Study the drawing (mm; zero at the part's minimum x, y, z) and answer. A direction names the side the tool comes from. Round coordinates to 2 decimals unless told otherwise and drop trailing zeros. Loops run counter-clockwise (first coordinate to the right, second up) from the corner with the lowest first, then second, coordinate; pieces in that order, holes last. Notation, with made-up numbers: (17.25, 24.5) -> (75.25, 24.5) arc R12 cw to (75.25, 38.5) -> close; hole circle Ø10 at (6.5, 56.25). An arc over 180 degrees is marked (long way). Use one line per item in the form item = value.
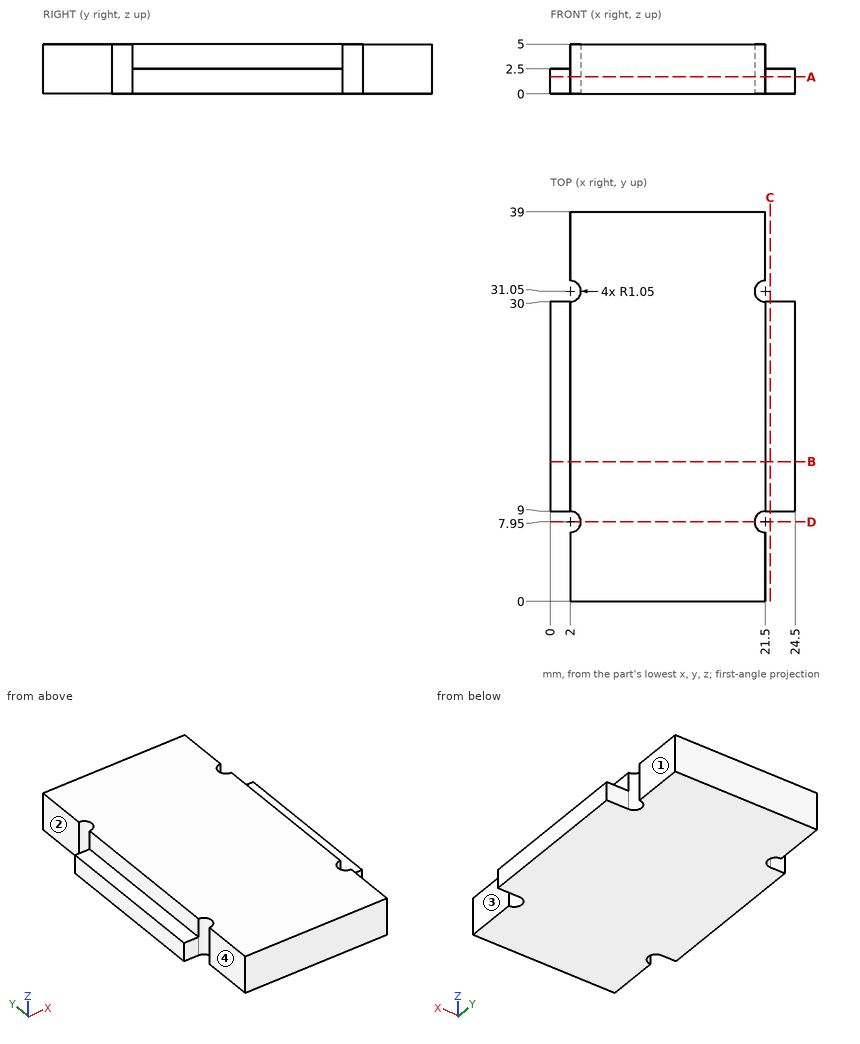
(1) Find section D-D, the plane y = 7.95. Write down the section's boundary in (x, z), then the cut area to 3 significant figures.
Completed:
outline = (3.05, 0) -> (20.45, 0) -> (20.45, 5) -> (3.05, 5) -> close
area = 87.0 mm2
(2) Given P1, Ø12, axis at x = 5.5, y = 24, coming from the -Z side; P2, Ø0.9, axis at x = 23.5, y = 15, coming from the +Z side; P3, Ø1.2, axis at x = 23.5, z = 1, coming from the -Y side; P4, Ø0.8, axis at y = 24, z = 3.5, coming from the +X side, each flat-ended and moving along its own axis, determine where each tip first touches the part or whether it passes through.
Completed:
P1 = 0
P2 = 2.5
P3 = 9
P4 = 21.5
(3) Find section A-A, the plane z = 1.7. Write down the section's boundary in (x, y), then the cut area to 3 significant figures.
Completed:
outline = (0, 9) -> (2, 9) arc R1.05 cw to (2, 6.9) -> (2, 0) -> (21.5, 0) -> (21.5, 6.9) arc R1.05 cw to (21.5, 9) -> (24.5, 9) -> (24.5, 30) -> (21.5, 30) arc R1.05 cw to (21.5, 32.1) -> (21.5, 39) -> (2, 39) -> (2, 32.1) arc R1.05 cw to (2, 30) -> (0, 30) -> close
area = 859 mm2
(4) For the marked faces 1, 2, 3 and 4, determine the directions among +Z, -Z, +X, -X, +Y, -Y from which every point of the face is accessible in a straight line to the end or side of a thin tool.
Completed:
face_1 = +Z, -Z, +X, +Y
face_2 = +Z, -Z, -X, +Y
face_3 = +Z, -Z, +X, -Y
face_4 = +Z, -Z, -X, -Y
(5) Find section C-C, the plane x = 22. Write down the section's boundary in (y, z).
Completed:
outline = (9, 0) -> (30, 0) -> (30, 2.5) -> (9, 2.5) -> close
(6) Consider L1, parallel to X at y = 23, z = 3.65; L2, parallel to Z at x = 21.75, y = 19; L3, parallel to X at y = 7, z = 4.2. Determine where each line is inside the solid, lowest interval first.
Completed:
L1 = 2 to 21.5
L2 = 0 to 2.5
L3 = 2.45 to 21.05
(7) Find section B-B, the plane y = 14. Write down the section's boundary in (x, z).
Completed:
outline = (0, 0) -> (24.5, 0) -> (24.5, 2.5) -> (21.5, 2.5) -> (21.5, 5) -> (2, 5) -> (2, 2.5) -> (0, 2.5) -> close
